Read the model definition and answer for the solid it produces. Units are mm, in the model's axes. A direction names the side the tool comes from. Coordinates: 2 decimals unless noted, no trailing zeros. Loops run counter-clockwise (first coordinate to the right, second up) from the corner with the lowest first, then second, coordinate; pieces in that order, holes last. Notation, with made-up numbers: (11, 31.5) -> (29, 31.5) arc R19 ccw to (29, 57.5) -> close; hole circle Ø8 at (73, 59.5). An arc over 180 degrees is marked (long way). Answer in a Markdown table with one row per item.
```python
from build123d import *

# Parameters (mm, degrees)
PAD029_DEPTH = 1.4
FILLET005_R  = 2
FILLET006_R  = 1


with BuildPart() as part:
    # Sketch046 → Pad029 (new body, symmetric)
    with BuildSketch(Plane.YZ):
        with BuildLine():
            Line((-25.701481, -40.1), (-24.051481, -40.1))
            Line((-24.051481, -29.1), (-24.051481, -40.1))
            ThreePointArc((-23.051481, -29.1), (-23.551481, -28.6), (-24.051481, -29.1))
            Line((-23.051481, -40.1), (-23.051481, -29.1))
            Line((-23.051481, -40.1), (-17.901481, -40.1))
            Line((-17.901481, -40.1), (-17.901481, -37.4))
            Line((-17.901481, -37.4), (-20.901481, -37.4))
            Line((-20.901481, -37.4), (-20.901481, -34.6))
            Line((-20.901481, -34.6), (-19.901481, -34.6))
            Line((-19.901481, -34.6), (-21.401481, -26.1))
            Line((-21.401481, -26.1), (-25.701481, -26.1))
            Line((-25.701481, -26.1), (-30.001481, -26.1))
            Line((-31.501481, -34.6), (-30.001481, -26.1))
            Line((-30.501481, -34.6), (-31.501481, -34.6))
            Line((-30.501481, -37.4), (-30.501481, -34.6))
            Line((-33.501481, -37.4), (-30.501481, -37.4))
            Line((-33.501481, -40.1), (-33.501481, -37.4))
            Line((-28.351481, -40.1), (-33.501481, -40.1))
            Line((-28.351481, -29.1), (-28.351481, -40.1))
            ThreePointArc((-27.351481, -29.1), (-27.851481, -28.6), (-28.351481, -29.1))
            Line((-27.351481, -40.1), (-27.351481, -29.1))
            Line((-25.701481, -40.1), (-27.351481, -40.1))
        make_face()
    extrude(amount=PAD029_DEPTH, both=True)

    # Fillet005
    fillet005_edges = [part.edges().sort_by_distance(p)[0] for p in [
        (0, -21.401481, -26.1),
        (0, -30.001481, -26.1),
    ]]
    fillet(fillet005_edges, radius=FILLET005_R)

    # Fillet006
    fillet006_edges = [part.edges().sort_by_distance(p)[0] for p in [
        (0, -33.501481, -40.1),
        (0, -17.901481, -40.1),
        (0, -28.351481, -40.1),
        (0, -27.351481, -40.1),
        (0, -24.051481, -40.1),
        (0, -23.051481, -40.1),
    ]]
    fillet(fillet006_edges, radius=FILLET006_R)


solid = part.part
```
1. Given pin 1 Ø0.8 at (x, z) = (0, -36) entering from +Y; pin 2 Ø1.4 at (x, z) = (0.5, -36) entering from -Y; pin 3 Ø0.8 at (x, z) = (-0.5, -32) entering from -Y, each flat-ended and moving along its own axis, determine where each tip first touches the part or whether it passes through.
A:
| item | result |
|---|---|
| pin 1 | stops at y = -20.9 |
| pin 2 | stops at y = -30.5 |
| pin 3 | stops at y = -31.11 |
2. A cutting plane is placed at C-C on z = -37.75. Give the vertices of the cut face in (x, y), and give its area (3 significant figures).
A:
| item | result |
|---|---|
| outline | (-1.4, -33.5) -> (1.4, -33.5) -> (1.4, -28.35) -> (-1.4, -28.35) -> close; (-1.4, -27.35) -> (1.4, -27.35) -> (1.4, -24.05) -> (-1.4, -24.05) -> close; (-1.4, -23.05) -> (1.4, -23.05) -> (1.4, -17.9) -> (-1.4, -17.9) -> close |
| area | 38.1 mm2 |
3. A tool of negligible diameter and unlimited length cuts with its end or side. For faces 4 (the flat face through (0, -20.4, -34.6)), 5 (the flat face through (-1.4, -26, -33)), 6 (the cylindrical face through (0.02, -33.216, -39.799)), 7 (the flat face through (0, -28.351, -34)), 8 (the flat face through (0, -32, -37.4)), from which of +Z, -Z, +X, -X, +Y, -Y can it reach the whole face along a straight path? Write none if from no direction.
A:
| item | result |
|---|---|
| face 4 | +X, -X, +Y |
| face 5 | +Z, -Z, -X, +Y, -Y |
| face 6 | -Z, +X, -X, -Y |
| face 7 | -Z, +X, -X |
| face 8 | +X, -X, -Y |
4. A cutting plane is placed at B-B on x = -1.05. Give the vertices of the cut face in (y, z).
A:
| item | result |
|---|---|
| outline | (-33.5, -39.1) arc R1 ccw to (-32.5, -40.1) -> (-29.35, -40.1) arc R1 ccw to (-28.35, -39.1) -> (-28.35, -29.1) arc R0.5 cw to (-27.35, -29.1) -> (-27.35, -39.1) arc R1 ccw to (-26.35, -40.1) -> (-25.05, -40.1) arc R1 ccw to (-24.05, -39.1) -> (-24.05, -29.1) arc R0.5 cw to (-23.05, -29.1) -> (-23.05, -39.1) arc R1 ccw to (-22.05, -40.1) -> (-18.9, -40.1) arc R1 ccw to (-17.9, -39.1) -> (-17.9, -37.4) -> (-20.9, -37.4) -> (-20.9, -34.6) -> (-19.9, -34.6) -> (-21.11, -27.75) arc R2 ccw to (-23.08, -26.1) -> (-28.32, -26.1) arc R2 ccw to (-30.29, -27.75) -> (-31.5, -34.6) -> (-30.5, -34.6) -> (-30.5, -37.4) -> (-33.5, -37.4) -> close |
5. The mould has two halves that part along Z. Classify faces 1 (the flat face through (0, -30.501, -36)), 2 (the flat face through (0, -20.5, -31.2)), 3 (the cylindrical face through (0.02, -28.65, -39.81)): pulls with the +Z half, pulls with the -Z half, needs draft (parallel to the pull), parting line crosses it, or undercut.
A:
| item | result |
|---|---|
| face 1 | undercut |
| face 2 | pulls with the +Z half |
| face 3 | pulls with the -Z half |
6. Find the intervals of material crossed by probe 1 along Y at (x, z) = (0, -35); probe 2 along Y at (x, z) = (0.15, -38); probe 3 along Z at (x, y) = (1.1, -25), in increasing order.
A:
| item | result |
|---|---|
| probe 1 | y = -30.5 to -28.35, -27.35 to -24.05, -23.05 to -20.9 |
| probe 2 | y = -33.5 to -28.35, -27.35 to -24.05, -23.05 to -17.9 |
| probe 3 | z = -40.1 to -26.1 |
7. A cutting plane is placed at A-A on z = -35. Give the vertices of the cut face in (x, y), and give its area (3 significant figures).
A:
| item | result |
|---|---|
| outline | (-1.4, -30.5) -> (1.4, -30.5) -> (1.4, -28.35) -> (-1.4, -28.35) -> close; (-1.4, -27.35) -> (1.4, -27.35) -> (1.4, -24.05) -> (-1.4, -24.05) -> close; (-1.4, -23.05) -> (1.4, -23.05) -> (1.4, -20.9) -> (-1.4, -20.9) -> close |
| area | 21.3 mm2 |
